```python
from build123d import *

# Parameters (mm, degrees)
BOSS_EXTRUDE1_DEPTH = 2.4
SKETCH2_R           = 1.5
BOSS_EXTRUDE2_DEPTH = 1.6
SKETCH3_W           = 8
SKETCH3_H           = 3.2
BOSS_EXTRUDE3_DEPTH = 1.6
SKETCH4_R           = 2.4
BOSS_EXTRUDE4_DEPTH = 1.8
SKETCH5_W           = 12.8
SKETCH5_H           = 4.8
CUT_EXTRUDE1_DEPTH  = 1.8
SKETCH6_R           = 1.6
BOSS_EXTRUDE5_DEPTH = 1.8


with BuildPart() as part:
    # Sketch1 → Boss-Extrude1 (new body)
    with BuildSketch(Plane.XY):
        with BuildLine():
            Line((9.6, 3.2), (0, 3.2))
            Line((0, 3.2), (0, 0))
            Line((0, 0), (12, 0))
            ThreePointArc((12, 0), (14, 4), (9.6, 3.2))
        make_face()
    extrude(amount=BOSS_EXTRUDE1_DEPTH)

    # Sketch2 → Boss-Extrude2 (add)
    with BuildSketch(Plane.XY.offset(2.4)):
        with Locations((12, 2.5)):
            Circle(SKETCH2_R)
    extrude(amount=BOSS_EXTRUDE2_DEPTH)

    # Sketch3 → Boss-Extrude3 (add)
    with BuildSketch(Plane.XY.offset(2.4)):
        with Locations((4, 1.6)):
            Rectangle(SKETCH3_W, SKETCH3_H)
    extrude(amount=BOSS_EXTRUDE3_DEPTH)

    # Mirror2: part across plane


with BuildPart() as part_1:
    add(part.part)
    add(part.part.mirror(Plane(origin=(12, 2.5, 4), x_dir=(1, 0, 0), z_dir=(0, 0, 1))))

    # Mirror3: part across plane


with BuildPart() as part_2:
    add(part_1.part)
    add(part_1.part.mirror(Plane(origin=(0, 3.2, 2.4), x_dir=(0, 0, 1), z_dir=(1, 0, 0))))

    # Sketch4 → Boss-Extrude4 (add)
    with BuildSketch(Plane(origin=(0, 3.2, 0), x_dir=(1, 0, 0), z_dir=(0, 1, 0))):
        with Locations((-4, -4)):
            Circle(SKETCH4_R)
        with Locations((4, -4)):
            Circle(SKETCH4_R)
    extrude(amount=BOSS_EXTRUDE4_DEPTH)

    # Sketch5 → Cut-Extrude1 (cut)
    with BuildSketch(Plane.XZ):
        with Locations((0, 4)):
            Rectangle(SKETCH5_W, SKETCH5_H)
    extrude(amount=-CUT_EXTRUDE1_DEPTH, mode=Mode.SUBTRACT)

    # Sketch6 → Boss-Extrude5 (add)
    with BuildSketch(Plane.XZ.offset(-1.8)):
        with Locations(Location((0, 4, 0), (0, 0, 270))):
            Circle(SKETCH6_R)
    extrude(amount=BOSS_EXTRUDE5_DEPTH)


solid = part_2.part
```
For this review, take the finished solid that the model builds, in its own axes (mm). A direction names the side the tool comes from. Coordinates: 2 decimals unless noted, no trailing zeros. Write each loop counter-clockwise with the first axis right and the second up, starting at its lowest first coordinate (ties: lowest second). Pieces come first, ordered by that corner, then holes.
(1) Tool access review of faces 1 (the face through (0, 1, 1.6)), 2 (the face through (-10, 2, 5.6)), 3 (the face through (0, 0, 1)), 4 (the face through (8, 2, 4)), 5 (the face through (6.29, 4.09, 3.28)): name each direction out of +Z, -Z, +X, -X, +Y, -Y from which nothing blocks a thin tool from reaching the whole face with its end or side.
(2) Add section D-D on y = 4.4. Give the boundary of the cut face in (x, z).
(3) Add section A-A on x = 9.25. Give the boundary of the cut face in (y, z), then the cut area to 3 significant figures.
(4) The part is to be moulded in two halves that separate along X. For faces 6 (the face through (0, 2, 0)), 7 (the face through (6.4, 1, 4)), 8 (the face through (10.8, 1.6, 4)), say which applies: +X half, -X half, draft (parallel to the pull), parting line (faces both ways), or undercut.
(5) Add section C-C on x = 4. Give the boundary of the cut face in (y, z).
(6) For pin 1 Ø2 at (x, y) = (2, 4.5) entering from -Z; pin 2 Ø2.5 at (y, z) = (1, 4.5) entering from -X; pin 3 Ø2 at (y, z) = (1.5, 5) entering from -X, all flat-tipped, find the tip position at first contact; note any pin that passes through.
(7) Wall thickness on probe 1 along Z at (x, y) = (1, 0.7); probe 2 along Z at (x, y) = (8.5, 2.2); probe 3 along Z at (x, y) = (3, 1.75): over which ranges is each line inside the solid? List them lowest first.
(8) Add section B-B on y = 2.5. Give the boundary of the cut face in (x, z), then the cut area to 3 significant figures.
Answer sheet:
1. face 1: -Y
1. face 2: none
1. face 3: +Z, -Z, +X, -X, -Y
1. face 4: +Y, -Y
1. face 5: +Y
2. outline: (-13.62, 0) - (-10.38, 0) - (-10.38, 2.4) - (-13.62, 2.4) - close; (-13.62, 5.6) - (-10.38, 5.6) - (-10.38, 8) - (-13.62, 8) - close; circle Ø4.8 at (-4, 4); circle Ø4.8 at (4, 4); (10.38, 0) - (13.62, 0) - (13.62, 2.4) - (10.38, 2.4) - close; (10.38, 5.6) - (13.62, 5.6) - (13.62, 8) - (10.38, 8) - close
3. outline: (0, 0) - (3.2, 0) - (3.2, 2.4) - (0, 2.4) - close; (0, 5.6) - (3.2, 5.6) - (3.2, 8) - (0, 8) - close
3. area: 15.4 mm2
4. face 6: draft
4. face 7: undercut
4. face 8: undercut
5. outline: (0, 0) - (3.2, 0) - (3.2, 1.6) - (5, 1.6) - (5, 6.4) - (3.2, 6.4) - (3.2, 8) - (0, 8) - (0, 6.4) - (1.8, 6.4) - (1.8, 1.6) - (0, 1.6) - close
6. pin 1: stops at z = 1.82
6. pin 2: stops at x = -14.33
6. pin 3: stops at x = -14.49
7. probe 1: z = 0 to 1.6, 2.75 to 5.25, 6.4 to 8
7. probe 2: z = 0 to 2.4, 5.6 to 8
7. probe 3: z = 0 to 1.6, 6.4 to 8
8. outline: (-14.5, 0) - (14.5, 0) - (14.5, 2.4) - (13.5, 2.4) - (13.5, 5.6) - (14.5, 5.6) - (14.5, 8) - (-14.5, 8) - (-14.5, 5.6) - (-13.5, 5.6) - (-13.5, 2.4) - (-14.5, 2.4) - close; hole (-10.5, 2.4) - (-8, 2.4) - (-8, 5.6) - (-10.5, 5.6) - close; hole (8, 2.4) - (10.5, 2.4) - (10.5, 5.6) - (8, 5.6) - close
8. area: 210 mm2
